Input: part model. Units: mm. Frame: model coordinates. Give positions to 0.01 mm unless a question says otherwise; leave off trailing zeros. Order: outer loops, then holes, each group sorted by start corner. A loop starts at its lowest first (then second) coordinate and runs counter-clockwise, first axis right, second up. Notation, with made-up numbers: M 88.5,-20.75 L 139.5,-20.75 A21 ccw 139.5,5.25 Z; hole C -12,88.5 d7. An arc over 180 degrees is marked long. Use a Markdown table: item, result.
Autodesk Inventor part; units mm, degrees
ref_plane "Work Plane1" through (0, 0, 6.35) normal (0, 0, 1) x (1, 0, 0)
ref_plane "Work Plane4" through (0, 19.1494, 6.35) normal (-1, 0, 0) x (0, -1, 0)
ref_plane "YZ Plane" through (0, 0, 0) normal (1, 0, 0) x (0, 1, 0)
sketch "Sketch1" plane through (0, 0, 0) normal (0, 0, 1) x (1, 0, 0)
  circle A0 centre (0, 0) radius 16.51
  circle A1 centre (0, 0) radius 20.32
  dimension "d0" = 40.64
  dimension "d2" = 33.02
extrude "Extrusion1" add sketch "Sketch1" along normal blind 11.43
sketch "Sketch2" plane through (0, 0, 11.43) normal (0, 0, 1) x (1, 0, 0)
  circle A0 centre (0, 0) radius 20.32
  circle A1 centre (0, 0) radius 15.875
  dimension "d5" = 31.75
extrude "Extrusion2" add sketch "Sketch2" along normal blind 1.27
fillet "Fillet1" radius 0.508 1 edges at (-15.875, 0, 11.43)
fillet "Fillet2" radius 0.508 1 edges at (-15.875, 0, 12.7)
ref_plane "Work Plane1" through (0, 0, 6.35) normal (0, 0, 1) x (1, 0, 0)
sketch "Sketch3" plane through (0, 0, 6.35) normal (0, 0, 1) x (1, 0, 0)
  line L0 (-20.32, 19.1494) -> (-20.32, -22.3588)
  circle A0 centre (0, 0) radius 20.32
  dimension "d11" = 20.32
sketch "Sketch4" plane through (0, 0, 12.7) normal (0, 0, 1) x (1, 0, 0)
  circle A0 centre (0, 0) radius 20.32
  circle A1 centre (0, 0) radius 16.383
ref_plane "Work Plane3" through (-20.32, 19.1494, 6.35) normal (-1, 0, 0) x (0, -1, 0)
ref_plane "Work Plane2" through (0, 0, 12.7) normal (0, 0, 1) x (1, 0, 0)
ref_plane "Work Plane4" through (0, 19.1494, 6.35) normal (-1, 0, 0) x (0, -1, 0)
sketch "Sketch6" plane through (0, 19.1494, 6.35) normal (-1, 0, 0) x (0, -1, 0)
  line L0 (39.364, 6.35) -> (35.554, 6.35)
  arc A0 (35.554, 6.35) -> (20.314, 11.4045) centre (19.0928, -17.78) ccw
  line L1 (39.364, 6.35) -> (39.364, 6.35)
  line L2 (31.744, 13.97) -> (20.314, 13.97)
  line L3 (20.314, 13.97) -> (20.314, 11.4045)
  arc A1 (39.364, 6.35) -> (31.744, 13.97) centre (31.744, 6.35) ccw
  line L4 (39.4694, 6.35) -> (-1.1706, 6.35)
  line L5 (19.044, 13.97) -> (19.044, 8.477)
  point P0 (19.1494, -6.35)
  point P1 (19.044, 5.9584)
  point P2 (19.044, 27.5056)
  point P3 (19.044, 11.43)
  point P4 (39.364, 13.97)
  dimension "d24" = 3.81
  dimension "d25" = 20.32
  dimension "d26" = 5.08
  dimension "d27" = 29.21
  dimension "d28" = 7.62
  dimension "d29" = 7.62
  dimension "d30" = 0
revolve "Revolution1" add sketch "Sketch6" angle 360 about axis through (0, 0.1054, 20.32) along (0, 0, -1)
sketch "Sketch7" plane through (0, 0.1054, 20.32) normal (0, 0, 1) x (1, 0, 0)
  circle A0 centre (0, 0) radius 1.27
  point P0 (0, -0.1054)
extrude "Extrusion3" add sketch "Sketch7" against normal blind 2.5654
sketch "Sketch8" plane through (0, 0.1054, 20.32) normal (0, 0, 1) x (1, 0, 0)
  circle A0 centre (0, 0) radius 12.7
  circle A1 centre (0, 0) radius 2.54
  circle A2 centre (0, 7.6441) radius 2.54
  point P0 (0, -0.1054)
  dimension "d34" = 5.08
  dimension "d36" = 5.08
extrude "Extrusion4" cut sketch "Sketch8" against normal blind 25.4 contours A1 | A2
properties part number "Motor End Cap" material "PVC-Piping"
1) Cut plane A-A on z = 4.5. Return loops of the section in (x, y).
Response values:
| item | result |
|---|---|
| outline | C 0,0 d40.64; hole C 0,0 d33.02 |
2) Material intervals for line 1 (Y direction, x = 0, z = 18.25); line 2 (Y direction, x = 0, z = 12.1) (3 decimals); line 3 (X direction, y = -12, z = 2.75), sorted ascending. Write a range as from..to.
Response values:
| item | result |
|---|---|
| line 1 | y = -17.82..-2.43, 2.65..5.21, 10.29..18.03 |
| line 2 | y = -20.32..-15.875, 15.875..20.32 |
| line 3 | x = -16.4..-11.34, 11.34..16.4 |
3) Mould query, pull axis X, two halves, no side actions, for faces 1 (the face through (-2.645, -20.147, 6.261)), 2 (the face through (-0.331, 10.268, 18.657)), 3 (the face through (15.748, -4.959, 5.635)), 4 (the face through (0, -3, 20.32)). Classes: released by +X, released by -X, zero draft, split by the parting line, or undercut.
Response values:
| item | result |
|---|---|
| face 1 | split by the parting line |
| face 2 | undercut |
| face 3 | undercut |
| face 4 | zero draft |
4) First-contact query: pin 1 Ø3 at (x, y) = (-7.5, 7) entering from -Z; pin 2 Ø2 at (x, z) = (-13, 17.5) entering from -Y; pin 3 Ø6 at (x, y) = (16, -5.5) entering from +Z. Flat tips, straight axial feed; report the tip coordinate or a pass-through.
Response values:
| item | result |
|---|---|
| pin 1 | stops at z = 15.36 |
| pin 2 | stops at y = -14.55 |
| pin 3 | stops at z = 20.22 |
5) Cut plane B-B on x = 0. State how many separate pieces and enclosed holes the cut face has, and give its area (3 significant figures).
Response values:
| item | result |
|---|---|
| separate pieces | 3 |
| enclosed holes | 0 |
| area | 238 mm² |
